Could you check a few things on this model? Use its own coordinates, in mm. A direction names the side the tool comes from. Coordinates: 2 decimals unless noted, no trailing zeros. Order: outer loops, then holes, each group sorted by start corner. A loop starts at its lowest first (then second) coordinate and runs counter-clockwise, first axis right, second up.
```python
from build123d import *

# Parameters (mm, degrees)
SKETCH1_W             = 120
SKETCH1_H             = 120
MAIN_BODY_DEPTH       = 150
HOLLOW_INSIDE_T       = -2
MAIN_PCB_HOLES_REACH  = 174.337
SKETCH2_R             = 1
LED_PCB_HOLES_REACH   = 174.337
SKETCH3_R             = 1.05
CONNECTOR_SLOTS_REACH = 174.337
SKETCH4_R             = 1.5
CUT_EXTRUDE1_DEPTH    = 4.75


with BuildPart() as part:
    # Sketch1 → Main-Body (new body)
    with BuildSketch(Plane(origin=(0, 0, 0), x_dir=(1, 0, 0), z_dir=(0, 1, 0))):
        Rectangle(SKETCH1_W, SKETCH1_H)
    extrude(amount=MAIN_BODY_DEPTH)

    # Hollow-Inside
    hollow_inside_openings = [part.faces().sort_by_distance(p)[0] for p in [
        (60, 75, 0),
    ]]
    offset(amount=HOLLOW_INSIDE_T, openings=hollow_inside_openings, kind=Kind.INTERSECTION)

    # Sketch2 → Main-PCB-Holes (cut, up to next)
    with BuildSketch(Plane.XZ, mode=Mode.PRIVATE) as main_pcb_holes_sk1:
        with Locations(Location((-40, 40, 0), (0, 0, 270))):
            Circle(SKETCH2_R)
    main_pcb_holes_tool1 = extrude(main_pcb_holes_sk1.sketch, amount=-MAIN_PCB_HOLES_REACH, mode=Mode.PRIVATE) & part.part
    # Sketch2 → Main-PCB-Holes (cut, up to next)
    with BuildSketch(Plane.XZ, mode=Mode.PRIVATE) as main_pcb_holes_sk2:
        with Locations(Location((40, 40, 0), (0, 0, 270))):
            Circle(SKETCH2_R)
    main_pcb_holes_tool2 = extrude(main_pcb_holes_sk2.sketch, amount=-MAIN_PCB_HOLES_REACH, mode=Mode.PRIVATE) & part.part
    # Sketch2 → Main-PCB-Holes (cut, up to next)
    with BuildSketch(Plane.XZ, mode=Mode.PRIVATE) as main_pcb_holes_sk3:
        with Locations(Location((40, -40, 0), (0, 0, 270))):
            Circle(SKETCH2_R)
    main_pcb_holes_tool3 = extrude(main_pcb_holes_sk3.sketch, amount=-MAIN_PCB_HOLES_REACH, mode=Mode.PRIVATE) & part.part
    # Sketch2 → Main-PCB-Holes (cut, up to next)
    with BuildSketch(Plane.XZ, mode=Mode.PRIVATE) as main_pcb_holes_sk4:
        with Locations(Location((-40, -40, 0), (0, 0, 270))):
            Circle(SKETCH2_R)
    main_pcb_holes_tool4 = extrude(main_pcb_holes_sk4.sketch, amount=-MAIN_PCB_HOLES_REACH, mode=Mode.PRIVATE) & part.part
    add(main_pcb_holes_tool1.solids().sort_by_distance((-40, 0, 40))[0], mode=Mode.SUBTRACT)
    add(main_pcb_holes_tool2.solids().sort_by_distance((40, 0, 40))[0], mode=Mode.SUBTRACT)
    add(main_pcb_holes_tool3.solids().sort_by_distance((40, 0, -40))[0], mode=Mode.SUBTRACT)
    add(main_pcb_holes_tool4.solids().sort_by_distance((-40, 0, -40))[0], mode=Mode.SUBTRACT)

    # Sketch3 → LED-PCB-Holes (cut, up to next)
    with BuildSketch(Plane(origin=(0, 150, 0), x_dir=(1, 0, 0), z_dir=(0, 1, 0)), mode=Mode.PRIVATE) as led_pcb_holes_sk1:
        with Locations(Location((-9, 5.23, 0), (0, 0, 270))):
            Circle(SKETCH3_R)
    led_pcb_holes_tool1 = extrude(led_pcb_holes_sk1.sketch, amount=-LED_PCB_HOLES_REACH, mode=Mode.PRIVATE) & part.part
    # Sketch3 → LED-PCB-Holes (cut, up to next)
    with BuildSketch(Plane(origin=(0, 150, 0), x_dir=(1, 0, 0), z_dir=(0, 1, 0)), mode=Mode.PRIVATE) as led_pcb_holes_sk2:
        with Locations(Location((9, 5.23, 0), (0, 0, 270))):
            Circle(SKETCH3_R)
    led_pcb_holes_tool2 = extrude(led_pcb_holes_sk2.sketch, amount=-LED_PCB_HOLES_REACH, mode=Mode.PRIVATE) & part.part
    # Sketch3 → LED-PCB-Holes (cut, up to next)
    with BuildSketch(Plane(origin=(0, 150, 0), x_dir=(1, 0, 0), z_dir=(0, 1, 0)), mode=Mode.PRIVATE) as led_pcb_holes_sk3:
        with Locations(Location((9, -2.27, 0), (0, 0, 270))):
            Circle(SKETCH3_R)
    led_pcb_holes_tool3 = extrude(led_pcb_holes_sk3.sketch, amount=-LED_PCB_HOLES_REACH, mode=Mode.PRIVATE) & part.part
    # Sketch3 → LED-PCB-Holes (cut, up to next)
    with BuildSketch(Plane(origin=(0, 150, 0), x_dir=(1, 0, 0), z_dir=(0, 1, 0)), mode=Mode.PRIVATE) as led_pcb_holes_sk4:
        with Locations(Location((-9, -2.27, 0), (0, 0, 270))):
            Circle(SKETCH3_R)
    led_pcb_holes_tool4 = extrude(led_pcb_holes_sk4.sketch, amount=-LED_PCB_HOLES_REACH, mode=Mode.PRIVATE) & part.part
    add(led_pcb_holes_tool1.solids().sort_by_distance((-9, 150, -5.23))[0], mode=Mode.SUBTRACT)
    add(led_pcb_holes_tool2.solids().sort_by_distance((9, 150, -5.23))[0], mode=Mode.SUBTRACT)
    add(led_pcb_holes_tool3.solids().sort_by_distance((9, 150, 2.27))[0], mode=Mode.SUBTRACT)
    add(led_pcb_holes_tool4.solids().sort_by_distance((-9, 150, 2.27))[0], mode=Mode.SUBTRACT)

    # Sketch4 → Connector-Slots (cut, up to next)
    with BuildSketch(Plane.XZ, mode=Mode.PRIVATE) as connector_slots_sk1:
        with Locations(Location((-12.5, 0, 0), (0, 0, 270))):
            Circle(SKETCH4_R)
    connector_slots_tool1 = extrude(connector_slots_sk1.sketch, amount=-CONNECTOR_SLOTS_REACH, mode=Mode.PRIVATE) & part.part
    # Sketch4 → Connector-Slots (cut, up to next)
    with BuildSketch(Plane.XZ, mode=Mode.PRIVATE) as connector_slots_sk2:
        with Locations(Location((12.5, 0, 0), (0, 0, 270))):
            Circle(SKETCH4_R)
    connector_slots_tool2 = extrude(connector_slots_sk2.sketch, amount=-CONNECTOR_SLOTS_REACH, mode=Mode.PRIVATE) & part.part
    # Sketch4 → Connector-Slots (cut, up to next)
    with BuildSketch(Plane.XZ, mode=Mode.PRIVATE) as connector_slots_sk3:
        with Locations(Location((-23.52, -15, 0), (0, 0, 270))):
            Circle(SKETCH4_R)
    connector_slots_tool3 = extrude(connector_slots_sk3.sketch, amount=-CONNECTOR_SLOTS_REACH, mode=Mode.PRIVATE) & part.part
    # Sketch4 → Connector-Slots (cut, up to next)
    with BuildSketch(Plane.XZ, mode=Mode.PRIVATE) as connector_slots_sk4:
        with Locations(Location((23.52, -15, 0), (0, 0, 270))):
            Circle(SKETCH4_R)
    connector_slots_tool4 = extrude(connector_slots_sk4.sketch, amount=-CONNECTOR_SLOTS_REACH, mode=Mode.PRIVATE) & part.part
    # Sketch4 → Connector-Slots (cut, up to next)
    with BuildSketch(Plane.XZ, mode=Mode.PRIVATE) as connector_slots_sk5:
        with Locations(Location((-23.52, 15, 0), (0, 0, 270))):
            Circle(SKETCH4_R)
    connector_slots_tool5 = extrude(connector_slots_sk5.sketch, amount=-CONNECTOR_SLOTS_REACH, mode=Mode.PRIVATE) & part.part
    # Sketch4 → Connector-Slots (cut, up to next)
    with BuildSketch(Plane.XZ, mode=Mode.PRIVATE) as connector_slots_sk6:
        with Locations(Location((23.52, 15, 0), (0, 0, 270))):
            Circle(SKETCH4_R)
    connector_slots_tool6 = extrude(connector_slots_sk6.sketch, amount=-CONNECTOR_SLOTS_REACH, mode=Mode.PRIVATE) & part.part
    # Sketch4 → Connector-Slots (cut, up to next)
    with BuildSketch(Plane.XZ, mode=Mode.PRIVATE) as connector_slots_sk7:
        with BuildLine():
            Line((-6.891594987, -5.117891943), (6.891594987, -5.117891943))
            ThreePointArc((6.891594987, -5.117891943), (8.211781315, -4.620259427), (8.875, -3.375))
            Line((8.875, -3.375), (9.75, 3.375))
            ThreePointArc((9.75, 3.375), (9.268962471, 4.952294386), (7.766594987, 5.632108057))
            Line((7.766594987, 5.632108057), (-7.766594987, 5.632108057))
            ThreePointArc((-7.766594987, 5.632108057), (-9.268962471, 4.952294386), (-9.75, 3.375))
            Line((-9.75, 3.375), (-8.875, -3.375))
            ThreePointArc((-8.875, -3.375), (-8.211781315, -4.620259427), (-6.891594987, -5.117891943))
        make_face()
    connector_slots_tool7 = extrude(connector_slots_sk7.sketch, amount=-CONNECTOR_SLOTS_REACH, mode=Mode.PRIVATE) & part.part
    # Sketch4 → Connector-Slots (cut, up to next)
    with BuildSketch(Plane.XZ, mode=Mode.PRIVATE) as connector_slots_sk8:
        with BuildLine():
            Line((-17.652212152, -20.046202025), (17.652212152, -20.046202025))
            ThreePointArc((17.652212152, -20.046202025), (18.944961945, -19.57224199), (19.625, -18.375))
            Line((19.625, -18.375), (20.75, -11.625))
            ThreePointArc((20.75, -11.625), (20.303252117, -10.003452233), (18.777212152, -9.296202025))
            Line((18.777212152, -9.296202025), (-18.777212152, -9.296202025))
            ThreePointArc((-18.777212152, -9.296202025), (-20.303252117, -10.003452233), (-20.75, -11.625))
            Line((-20.75, -11.625), (-19.625, -18.375))
            ThreePointArc((-19.625, -18.375), (-18.944961945, -19.57224199), (-17.652212152, -20.046202025))
        make_face()
    connector_slots_tool8 = extrude(connector_slots_sk8.sketch, amount=-CONNECTOR_SLOTS_REACH, mode=Mode.PRIVATE) & part.part
    # Sketch4 → Connector-Slots (cut, up to next)
    with BuildSketch(Plane.XZ, mode=Mode.PRIVATE) as connector_slots_sk9:
        with BuildLine():
            Line((-17.652212152, 9.953797975), (17.652212152, 9.953797975))
            ThreePointArc((17.652212152, 9.953797975), (18.944961945, 10.42775801), (19.625, 11.625))
            Line((19.625, 11.625), (20.75, 18.375))
            ThreePointArc((20.75, 18.375), (20.303252117, 19.996547767), (18.777212152, 20.703797975))
            Line((18.777212152, 20.703797975), (-18.777212152, 20.703797975))
            ThreePointArc((-18.777212152, 20.703797975), (-20.303252117, 19.996547767), (-20.75, 18.375))
            Line((-20.75, 18.375), (-19.625, 11.625))
            ThreePointArc((-19.625, 11.625), (-18.944961945, 10.42775801), (-17.652212152, 9.953797975))
        make_face()
    connector_slots_tool9 = extrude(connector_slots_sk9.sketch, amount=-CONNECTOR_SLOTS_REACH, mode=Mode.PRIVATE) & part.part
    add(connector_slots_tool1.solids().sort_by_distance((-12.5, 0, 0))[0], mode=Mode.SUBTRACT)
    add(connector_slots_tool2.solids().sort_by_distance((12.5, 0, 0))[0], mode=Mode.SUBTRACT)
    add(connector_slots_tool3.solids().sort_by_distance((-23.52, 0, -15))[0], mode=Mode.SUBTRACT)
    add(connector_slots_tool4.solids().sort_by_distance((23.52, 0, -15))[0], mode=Mode.SUBTRACT)
    add(connector_slots_tool5.solids().sort_by_distance((-23.52, 0, 15))[0], mode=Mode.SUBTRACT)
    add(connector_slots_tool6.solids().sort_by_distance((23.52, 0, 15))[0], mode=Mode.SUBTRACT)
    add(connector_slots_tool7.solids().sort_by_distance((0, 0, 0.368259))[0], mode=Mode.SUBTRACT)
    add(connector_slots_tool8.solids().sort_by_distance((0, 0, -14.605881))[0], mode=Mode.SUBTRACT)
    add(connector_slots_tool9.solids().sort_by_distance((0, 0, 15.394119))[0], mode=Mode.SUBTRACT)

    # Sketch12 → Cut-Extrude1 (cut, symmetric)
    with BuildSketch(Plane(origin=(0, 75, 0), x_dir=(1, 0, 0), z_dir=(0, 1, 0))):
        Polygon((30.88, 60), (29.88, 60), (29.88, 59.702820323), (28.68, 59.01), (28.68, 58), (30.88, 58), (31, 58), (31, 60), align=None)
    cut_extrude1 = extrude(amount=CUT_EXTRUDE1_DEPTH, both=True, mode=Mode.SUBTRACT)

    # Mirror1: Cut-Extrude1 across plane
    add(cut_extrude1.mirror(Plane.XY), mode=Mode.SUBTRACT)


solid = part.part
```
Item 1: Suppose I cut it at A-A (x = -37). List the corners of the cut face in (y, z) for me.
Item 2: Suppose I cut it at B-B (y = 99). List the corners of the cut face in (x, z) for me, and give its area (3 significant figures).
Item 3: Suppose I cut it at C-C (z = -44). List the corners of the cut face in (x, y) for me, and give its area (3 significant figures).
Item 4: For pin 1 Ø4 at (y, z) = (121.5, -7.5) entering from +X; pin 2 Ø1.8 at (x, z) = (-23.52, 15) entering from -Y, each with a flat end and sliding along its axis, tell me the tip position at first contact or that it passes through.
Item 5: Thinking about a two-plate mould opening in Y: for faces 1 (the face through (0, 148, -1)), 2 (the face through (-1, 150, -1)), 3 (the face through (-58, 74, 1)), 4 (the face through (-1, 74, -60)), which applies, +Y half, -Y half, draft (parallel to the pull), parting line (faces both ways), or undercut?
Item 6: Which directions (+Z, -Z, +X, -X, +Y, -Y) give clear straight access to the entire face, cutting with the end or side of a thin tool? Please do faces 5 (the face through (-1, 74, 60)), 6 (the face through (0, 74, -58)).
Item 7: I need wall thicknesses on line 1 (Y direction, x = 5, z = 9.5); line 2 (Z direction, x = -29, y = 82); line 3 (X direction, y = 1, z = 0). Which ranges of each line are inside material? Lowest first, please.
Geometry results:
1. outline: (0, -60) - (150, -60) - (150, 60) - (0, 60) - close; hole (2, -58) - (148, -58) - (148, 58) - (2, 58) - close
2. outline: (-60, -60) - (60, -60) - (60, -58) - (-58, -58) - (-58, 58) - (60, 58) - (60, 60) - (-60, 60) - close
2. area: 712 mm2
3. outline: (-60, 0) - (60, 0) - (60, 2) - (-58, 2) - (-58, 148) - (60, 148) - (60, 150) - (-60, 150) - close
3. area: 772 mm2
4. pin 1: stops at x = -58
4. pin 2: stops at y = 148
5. face 1: undercut
5. face 2: +Y half
5. face 3: undercut
5. face 4: draft
6. face 5: +Z, +X, -X, +Y, -Y
6. face 6: +X
7. line 1: y = 0 to 2, 148 to 150
7. line 2: z = -60 to -58, 58 to 60
7. line 3: x = -60 to -14, -11 to -9.31, 9.31 to 11, 14 to 60
